Design review of the part built by this model. Coordinates are the model's own, in mm. Round coordinates to 2 decimals unless told otherwise and drop trailing zeros. Loops run counter-clockwise (first coordinate to the right, second up) from the corner with the lowest first, then second, coordinate; pieces in that order, holes last. Notation, with made-up numbers: (31.5, 0) - (72.5, 0) arc R15 cw to (72.5, 14) - close; hole circle Ø1 at (63.25, -10). An arc over 180 degrees is marked (long way). Return JSON: item names as keys, results as strings. Group by question number.
from build123d import *

# Parameters (mm, degrees)
CLEVIS_START = -4e-06
SKETCH6_R    = 4.05
CLEVIS_DEPTH = 5.00001


with BuildPart() as part:
    # Sketch5 → Body (revolve)
    with BuildSketch(Plane.XY):
        with BuildLine():
            Line((5, 496.16336506), (5, -5))
            Line((5, -5), (0, -5))
            Line((0, -5), (0, 500))
            ThreePointArc((0, 500), (3.151181035, 498.930318177), (5, 496.16336506))
        make_face()
    revolve(axis=Axis((0, -5, 0), (0, 1, 0)))

    # Sketch6 → Clevis (add)
    with BuildSketch(Plane.XY.offset(-2.5).offset(CLEVIS_START)):
        with BuildLine():
            Line((-7.5, 515), (-7.5, 496.16336506))
            ThreePointArc((-7.5, 496.16336506), (0, 491.912847956), (7.5, 496.16336506))
            Line((7.5, 496.16336506), (7.5, 515))
            ThreePointArc((7.5, 515), (0, 522.5), (-7.5, 515))
        make_face()
        with Locations((0, 515)):
            Circle(SKETCH6_R, mode=Mode.SUBTRACT)
    extrude(amount=CLEVIS_DEPTH)


solid = part.part
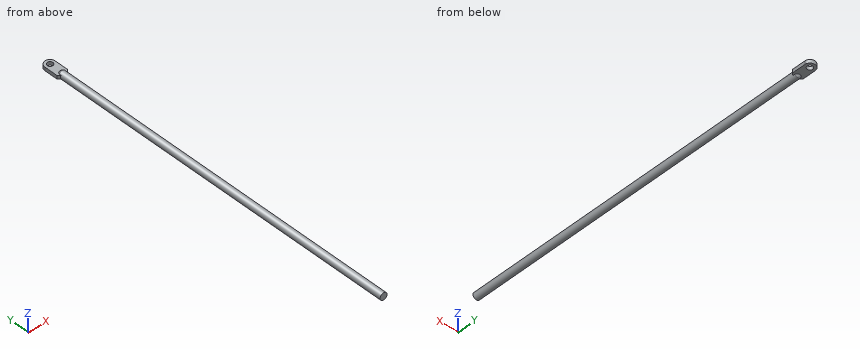
Q1. Insertion check: pin 1 Ø7.5 at (x, y) = (-2, 511.5) entering from +Z; pin 2 Ø2 at (x, y) = (-3.5, 232.5) entering from -Z; pin 3 Ø1 at (x, y) = (5, 208) entering from +Z. Each pin has a flat end and moves straight along its axis. Give the tip position at first contact, or say it passes through.
Q2. Add section C-C, the plane y = 237. State the section outline as (x, z) points, plus the area to 3 significant figures.
Q3. For line 1 (X direction, y = 515, z = -1.1); line 2 (Y direction, x = 0, z = -0.35); line 3 (X direction, y = 78.5, z = 0.75), list the stretches that pass through material, from the lowest coordinate up.
Q4. Add section A-A, the plane x = 0. State the section outline as (y, z) points.
Q5. Add section B-B, the plane z = 0. State the section outline as (x, y) points.
Evaluation:
{
 "1": {"pin 1": "z = 2.5", "pin 2": "z = -4.33", "pin 3": "z = 2.18"},
 "2": {"outline": "circle Ø10 at (0, 0)", "area": "78.5 mm²"},
 "3": {"line 1": "-7.5 to -4.05, 4.05 to 7.5", "line 2": "-5 to 510.95, 519.05 to 522.5", "line 3": "-4.94 to 4.94"},
 "4": {"outline": "(-5, -5) - (496.16, -5) arc R5.18 ccw to (499.36, -2.5) - (510.95, -2.5) - (510.95, 2.5) - (499.36, 2.5) arc R5.18 ccw to (496.16, 5) - (-5, 5) - close; (519.05, -2.5) - (522.5, -2.5) - (522.5, 2.5) - (519.05, 2.5) - close"},
 "5": {"outline": "(-7.5, 496.16) arc R8.74 ccw to (-5, 493.48) - (-5, -5) - (5, -5) - (5, 493.48) arc R8.74 ccw to (7.5, 496.16) - (7.5, 515) arc R7.5 ccw to (-7.5, 515) - close; hole circle Ø8.1 at (0, 515)"}
}
